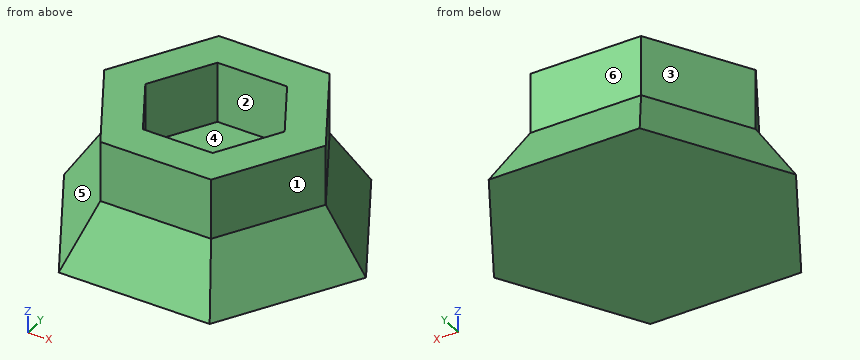
from build123d import *

# Parameters (mm, degrees)
BOSS_EXTRUDE1_DEPTH = 5
BOSS_EXTRUDE2_DEPTH = 5
BOSS_EXTRUDE2_DRAFT = 30


with BuildPart() as part:
    # Sketch1 → Boss-Extrude1 (new body)
    with BuildSketch(Plane.XY):
        Polygon((9.17986928, 0), (4.58993464, 7.95), (-4.58993464, 7.95), (-9.17986928, 0), (-4.58993464, -7.95), (4.58993464, -7.95), align=None)
        Polygon((5.773502692, 0), (2.886751346, 5), (-2.886751346, 5), (-5.773502692, 0), (-2.886751346, -5), (2.886751346, -5), align=None, mode=Mode.SUBTRACT)
    extrude(amount=BOSS_EXTRUDE1_DEPTH)


with BuildPart() as boss_extrude2_tool:
    # Sketch1_2 → Boss-Extrude2 (with draft: the straight prism first)
    with BuildSketch(Plane.XY):
        Polygon((9.17986928, 0), (4.58993464, 7.95), (-4.58993464, 7.95), (-9.17986928, 0), (-4.58993464, -7.95), (4.58993464, -7.95), align=None)
    extrude(amount=-BOSS_EXTRUDE2_DEPTH)
    # Boss-Extrude2: the draft: its side faces are tilted about the plane it starts from
    boss_extrude2_sides = [boss_extrude2_tool.faces().sort_by_distance(p)[0] for p in [
        (6.88490196, 3.975, -2.5),
        (0, 7.95, -2.5),
        (-6.88490196, 3.975, -2.5),
        (-6.88490196, -3.975, -2.5),
        (0, -7.95, -2.5),
        (6.88490196, -3.975, -2.5),
    ]]
    draft(boss_extrude2_sides, Plane.XY, BOSS_EXTRUDE2_DRAFT)


with BuildPart() as part_1:
    add(part.part)

    # Boss-Extrude2: add boss_extrude2_tool
    add(boss_extrude2_tool.part)


solid = part_1.part
Can you work these out from the model? Positions are in its coordinate system, mm. Face numbers are marked on the shaded views. A direction names the side the tool comes from. Coordinates: 2 decimals unless noted, no trailing zeros. Loops run counter-clockwise (first coordinate to the right, second up) from the corner with the lowest first, then second, coordinate; pieces in that order, holes last. Notation, with made-up numbers: M 0,-20.75 L 13,-20.75 A20 cw 13,3.25 Z; hole C 25.25,83.25 d8. An arc over 180 degrees is marked long. Answer as CSV lines item,"result". Start each with the question number.
1. Suppose I cut it at C-C, the plane y = 1.5. List the corners of the cut face in (x, z) for me.
2. Suppose I cut it at A-A, the plane z = 1.5. List the corners of the cut face in (x, y) for me.
3. If I drill on probe 1 along Z at (x, y) = (1.25, -3.5); probe 2 along X at (y, z) = (2, 2); probe 3 along X at (y, z) = (-1, 4), over which ranges is the centre line in solid material (lowest first)? Write a range as [from, to].
4. For pin 1 Ø2.5 at (x, z) = (-0.5, 3) entering from -Y; pin 2 Ø2.5 at (x, z) = (0, 2) entering from +Y; pin 3 Ø6 at (y, z) = (-8.5, 2.5) entering from +X, each with a flat end and sliding along its axis, tell me the tip position at first contact or that it passes through.
5. Thinking about a two-plate mould opening in X: for the marked faces 4, 5 and 6, which applies, +X half, -X half, draft (parallel to the pull), parting line (faces both ways), or undercut?
6. For the marked faces 1, 2 and 3, which set-ups out of +Z, -Z, +X, -X, +Y, -Y let a thin tool reach every point of the face, with its end or its side?
7. Suppose I cut it at D-D, the plane z = -1.75. List the corners of the cut face in (x, y) for me.
8. Suppose I cut it at B-B, the plane x = 1. List the corners of the cut face in (y, z) for me.
Output:
1,outline,"M -11.65,-5 L 11.65,-5 L 8.31,0 L 8.31,5 L 4.91,5 L 4.91,0 L -4.91,0 L -4.91,5 L -8.31,5 L -8.31,0 Z"
2,outline,"M -9.18,0 L -4.59,-7.95 L 4.59,-7.95 L 9.18,0 L 4.59,7.95 L -4.59,7.95 Z; hole M -5.77,0 L -2.89,-5 L 2.89,-5 L 5.77,0 L 2.89,5 L -2.89,5 Z"
3,probe 1,"z = [-5, 0]"
3,probe 2,"x = [-8.03, -4.62], [4.62, 8.03]"
3,probe 3,"x = [-8.6, -5.2], [5.2, 8.6]"
4,pin 1,"stops at y = -7.95"
4,pin 2,"stops at y = 7.95"
4,pin 3,"stops at x = 6"
5,face 4,"undercut"
5,face 5,"-X half"
5,face 6,"draft"
6,face 1,"+Z, +X, -Y"
6,face 2,"+Z"
6,face 3,"+Z, -X, +Y"
7,outline,"M -10.35,0 L -5.17,-8.96 L 5.17,-8.96 L 10.35,0 L 5.17,8.96 L -5.17,8.96 Z"
8,outline,"M -10.84,-5 L 10.84,-5 L 7.95,0 L 7.95,5 L 5,5 L 5,0 L -5,0 L -5,5 L -7.95,5 L -7.95,0 Z"
